from build123d import *

# Parameters (mm, degrees)
BOSS_EXTRUDE1_DEPTH  = 4
BOSS_EXTRUDE1_DRAFT  = -1
SHELL1_T             = -0.35
SKETCH2_W            = 12.58
SKETCH2_H            = 6.98
CUT_EXTRUDE1_DEPTH   = 2
SKETCH3_W            = 13.5
SKETCH3_H            = 13.096235698
CUT_EXTRUDE2_DEPTH   = 0.2
BOSS_EXTRUDE3_REACH  = 20.425
BOSS_EXTRUDE4_REACH  = 20.425
LPATTERN2_COUNT      = 2
LPATTERN2_PITCH      = 4
MIRROR4_COPY_1_REACH = 20.425
LPATTERN3_COUNT      = 2
LPATTERN3_PITCH      = 4
MIRROR5_COPY_1_REACH = 20.425
BOSS_EXTRUDE5_REACH  = 18.785
LPATTERN4_COUNT      = 2
LPATTERN4_PITCH      = 5
MIRROR6_COPY_1_REACH = 18.785
MIRROR6_COPY_2_REACH = 18.785


with BuildPart() as part:
    # Sketch1 → Boss-Extrude1 (with draft: the straight prism first)
    with BuildSketch(Plane(origin=(0, 0, 0), x_dir=(1, 0, 0), z_dir=(0, 1, 0))):
        with BuildLine():
            Line((-7.5, -8.5), (7.5, -8.5))
            ThreePointArc((7.5, -8.5), (8.207106781, -8.207106781), (8.5, -7.5))
            Line((8.5, -7.5), (8.5, 7.5))
            ThreePointArc((8.5, 7.5), (8.207106781, 8.207106781), (7.5, 8.5))
            Line((7.5, 8.5), (-7.5, 8.5))
            ThreePointArc((-7.5, 8.5), (-8.207106781, 8.207106781), (-8.5, 7.5))
            Line((-8.5, 7.5), (-8.5, -7.5))
            ThreePointArc((-8.5, -7.5), (-8.207106781, -8.207106781), (-7.5, -8.5))
        make_face()
    extrude(amount=-BOSS_EXTRUDE1_DEPTH)
    # Boss-Extrude1: the draft: its side faces are tilted about the plane it starts from
    boss_extrude1_sides = [part.faces().sort_by_distance(p)[0] for p in [
        (0, -2, 8.5),
        (8.207106781, -2, 8.207106781),
        (8.5, -2, 0),
        (8.207106781, -2, -8.207106781),
        (0, -2, -8.5),
        (-8.207106781, -2, -8.207106781),
        (-8.5, -2, 0),
        (-8.207106781, -2, 8.207106781),
    ]]
    draft(boss_extrude1_sides, Plane(origin=(0, 0, 0), x_dir=(1, 0, 0), z_dir=(0, 1, 0)), BOSS_EXTRUDE1_DRAFT)

    # Shell1
    shell1_openings = [part.faces().sort_by_distance(p)[0] for p in [
        (0, 0, 0),
    ]]
    offset(amount=SHELL1_T, openings=shell1_openings, kind=Kind.INTERSECTION)

    # Sketch2 → Cut-Extrude1 (cut)
    with BuildSketch(Plane.XZ.offset(4)):
        with Locations((0, 1.01)):
            Rectangle(SKETCH2_W, SKETCH2_H)
    extrude(amount=-CUT_EXTRUDE1_DEPTH, mode=Mode.SUBTRACT)

    # Sketch3 → Cut-Extrude2 (cut)
    with BuildSketch(Plane(origin=(0, -3.65, 0), x_dir=(1, 0, 0), z_dir=(0, 1, 0))):
        with Locations((0, 1.238117849)):
            Rectangle(SKETCH3_W, SKETCH3_H)
    extrude(amount=-CUT_EXTRUDE2_DEPTH, mode=Mode.SUBTRACT)

    # Boss-Extrude3: up to this plane
    boss_extrude3_end = Plane(origin=(8.150053307, 0.006108342, 7.5), z_dir=(0.9998476951563913, -0.01745240643728355, 0))
    # Sketch11 → Boss-Extrude3 (add, up to the surface)
    with BuildSketch(Plane.ZY.offset(-7.35), mode=Mode.PRIVATE) as boss_extrude3_sk1:
        Polygon((-0.455489584, -1.1), (0.46508987, -1.1), (0.509600286, -3.65), (-0.5, -3.65), align=None)
    boss_extrude3_tool1 = split(extrude(boss_extrude3_sk1.sketch, amount=-BOSS_EXTRUDE3_REACH, mode=Mode.PRIVATE), bisect_by=boss_extrude3_end, keep=Keep.BOTH, mode=Mode.PRIVATE)
    boss_extrude3 = boss_extrude3_tool1.solids().sort_by_distance((7.35, -2.394601, 0.0048))[0]
    add(boss_extrude3)

    # Boss-Extrude4: up to this plane
    boss_extrude4_end = Plane(origin=(-8.150053307, 0.006108342, 7.5), z_dir=(-0.9998476951563913, -0.01745240643728355, 0))
    # Sketch13 → Boss-Extrude4 (add, up to the surface)
    with BuildSketch(Plane(origin=(-7.35, 0, 0), x_dir=(0, 0, -1), z_dir=(1, 0, 0)), mode=Mode.PRIVATE) as boss_extrude4_sk1:
        Polygon((-0.5, -3.65), (0.509600286, -3.65), (0.46508987, -1.1), (-0.455489584, -1.1), align=None)
    boss_extrude4_tool1 = split(extrude(boss_extrude4_sk1.sketch, amount=-BOSS_EXTRUDE4_REACH, mode=Mode.PRIVATE), bisect_by=boss_extrude4_end, keep=Keep.BOTH, mode=Mode.PRIVATE)
    boss_extrude4 = boss_extrude4_tool1.solids().sort_by_distance((-7.35, -2.394601, -0.0048))[0]
    add(boss_extrude4)

    # LPattern2: Boss-Extrude3 ×2
    with Locations(*[(0, 0, i * LPATTERN2_PITCH) for i in range(1, LPATTERN2_COUNT)]):
        add(boss_extrude3)

    # Mirror4: Boss-Extrude3 across plane
    add(boss_extrude3.mirror(Plane.XY))

    # Mirror4 copy 1: up to this plane
    mirror4_copy_1_end = Plane(origin=(8.150053307, 0.006108342, 7.5), z_dir=(0.9998476951563913, -0.01745240643728355, 0))
    # Mirror4 copy 1 sketch → Mirror4 copy 1 (add, up to the surface)
    with BuildSketch(Plane(origin=(7.35, 0, -4), x_dir=(0, 0, -1), z_dir=(-1, 0, 0)), mode=Mode.PRIVATE) as mirror4_copy_1_sk1:
        Polygon((-0.455489584, 1.1), (0.46508987, 1.1), (0.509600286, 3.65), (-0.5, 3.65), align=None)
    mirror4_copy_1_tool1 = split(extrude(mirror4_copy_1_sk1.sketch, amount=-MIRROR4_COPY_1_REACH, mode=Mode.PRIVATE), bisect_by=mirror4_copy_1_end, keep=Keep.BOTH, mode=Mode.PRIVATE)
    add(mirror4_copy_1_tool1.solids().sort_by_distance((7.35, -2.394601, 0.0048))[0])

    # LPattern3: Boss-Extrude4 ×2
    with Locations(*[(0, 0, i * LPATTERN3_PITCH) for i in range(1, LPATTERN3_COUNT)]):
        add(boss_extrude4)

    # Mirror5: Boss-Extrude4 across plane
    add(boss_extrude4.mirror(Plane.XY))

    # Mirror5 copy 1: up to this plane
    mirror5_copy_1_end = Plane(origin=(-8.150053307, 0.006108342, 7.5), z_dir=(-0.9998476951563913, -0.01745240643728355, 0))
    # Mirror5 copy 1 sketch → Mirror5 copy 1 (add, up to the surface)
    with BuildSketch(Plane(origin=(-7.35, 0, -4), x_dir=(0, 0, 1), z_dir=(1, 0, 0)), mode=Mode.PRIVATE) as mirror5_copy_1_sk1:
        Polygon((-0.5, 3.65), (0.509600286, 3.65), (0.46508987, 1.1), (-0.455489584, 1.1), align=None)
    mirror5_copy_1_tool1 = split(extrude(mirror5_copy_1_sk1.sketch, amount=-MIRROR5_COPY_1_REACH, mode=Mode.PRIVATE), bisect_by=mirror5_copy_1_end, keep=Keep.BOTH, mode=Mode.PRIVATE)
    add(mirror5_copy_1_tool1.solids().sort_by_distance((-7.35, -2.394601, -0.0048))[0])

    # Boss-Extrude5: up to this plane
    boss_extrude5_end = Plane(origin=(-7.5, 0.006108342, 8.150053307), z_dir=(0, -0.017452406437283553, 0.9998476951563913))
    # Sketch16 → Boss-Extrude5 (add, up to the surface)
    with BuildSketch(Plane.XY.offset(5.41), mode=Mode.PRIVATE) as boss_extrude5_sk1:
        Polygon((-0.5, -3.65), (0.5, -3.65), (0.455489584, -1.1), (-0.455489584, -1.1), align=None)
    boss_extrude5_tool1 = split(extrude(boss_extrude5_sk1.sketch, amount=BOSS_EXTRUDE5_REACH, mode=Mode.PRIVATE), bisect_by=boss_extrude5_end, keep=Keep.BOTH, mode=Mode.PRIVATE)
    boss_extrude5 = boss_extrude5_tool1.solids().sort_by_distance((0, -2.394798, 5.41))[0]
    add(boss_extrude5)

    # LPattern4: Boss-Extrude5 ×2
    with Locations(*[(i * LPATTERN4_PITCH, 0, 0) for i in range(1, LPATTERN4_COUNT)]):
        add(boss_extrude5)

    # Mirror6 copy 1: up to this plane
    mirror6_copy_1_end = Plane(origin=(-7.5, 0.006108342, 8.150053307), z_dir=(0, -0.017452406437283553, 0.9998476951563913))
    # Mirror6 copy 1 sketch → Mirror6 copy 1 (add, up to the surface)
    with BuildSketch(Plane(origin=(-5, 0, 5.41), x_dir=(-1, 0, 0), z_dir=(0, 0, 1)), mode=Mode.PRIVATE) as mirror6_copy_1_sk1:
        Polygon((-0.5, 3.65), (0.5, 3.65), (0.455489584, 1.1), (-0.455489584, 1.1), align=None)
    mirror6_copy_1_tool1 = split(extrude(mirror6_copy_1_sk1.sketch, amount=MIRROR6_COPY_1_REACH, mode=Mode.PRIVATE), bisect_by=mirror6_copy_1_end, keep=Keep.BOTH, mode=Mode.PRIVATE)
    add(mirror6_copy_1_tool1.solids().sort_by_distance((0, -2.394798, 5.41))[0])

    # Mirror6 copy 2: up to this plane
    mirror6_copy_2_end = Plane(origin=(-7.5, 0.006108342, 8.150053307), z_dir=(0, -0.017452406437283553, 0.9998476951563913))
    # Mirror6 copy 2 sketch → Mirror6 copy 2 (add, up to the surface)
    with BuildSketch(Plane(origin=(0, 0, 5.41), x_dir=(-1, 0, 0), z_dir=(0, 0, 1)), mode=Mode.PRIVATE) as mirror6_copy_2_sk1:
        Polygon((-0.5, 3.65), (0.5, 3.65), (0.455489584, 1.1), (-0.455489584, 1.1), align=None)
    mirror6_copy_2_tool1 = split(extrude(mirror6_copy_2_sk1.sketch, amount=MIRROR6_COPY_2_REACH, mode=Mode.PRIVATE), bisect_by=mirror6_copy_2_end, keep=Keep.BOTH, mode=Mode.PRIVATE)
    add(mirror6_copy_2_tool1.solids().sort_by_distance((0, -2.394798, 5.41))[0])

    # Sweep1: sweep along a path in Sketch18
    with BuildLine(Plane(origin=(0, -2, 0), x_dir=(-1, 0, 0), z_dir=(0, -1, 0))) as sweep1_path:
        Line((8.5, 7.5), (8.5, -7.5))
        ThreePointArc((8.5, -7.5), (8.207106781, -8.207106781), (7.5, -8.5))
        Line((7.5, -8.5), (-7.5, -8.5))
        ThreePointArc((-7.5, -8.5), (-8.207106781, -8.207106781), (-8.5, -7.5))
        Line((-8.5, -7.5), (-8.5, 7.5))
        ThreePointArc((-8.5, 7.5), (-8.207106781, 8.207106781), (-7.5, 8.5))
        Line((-7.5, 8.5), (7.5, 8.5))
        ThreePointArc((7.5, 8.5), (8.207106781, 8.207106781), (8.5, 7.5))
    # Sketch17 → Sweep1 (sweep)
    with BuildSketch(Plane.XY):
        Polygon((-8.5, 0), (-8.46508987, -2), (-8.76508987, -2), align=None)
    sweep(path=sweep1_path.line)

    # Sweep2: sweep along a path in Sketch23
    with BuildLine(Plane(origin=(0, 0, 0), x_dir=(1, 0, 0), z_dir=(0, 1, 0))) as sweep2_path:
        Line((8.149946685, -7.5), (8.149946685, 7.5))
        ThreePointArc((8.149946685, 7.5), (7.959581709, 7.959581709), (7.5, 8.149946685))
        Line((7.5, 8.149946685), (-7.5, 8.149946685))
        ThreePointArc((-7.5, 8.149946685), (-7.959581709, 7.959581709), (-8.149946685, 7.5))
        Line((-8.149946685, 7.5), (-8.149946685, -7.5))
        ThreePointArc((-8.149946685, -7.5), (-7.959581709, -7.959581709), (-7.5, -8.149946685))
        Line((-7.5, -8.149946685), (7.5, -8.149946685))
        ThreePointArc((7.5, -8.149946685), (7.959581709, -7.959581709), (8.149946685, -7.5))
    # Sketch19 → Sweep2 (sweep)
    with BuildSketch(Plane.XY):
        Polygon((8.149946685, 0), (8.148156734, -0.102546259), (8.14097505, -0.102546259), align=None)
    sweep(path=sweep2_path.line)


solid = part.part
Could you check a few things on this model? Use its own coordinates, in mm. A direction names the side the tool comes from. Coordinates: 2 decimals unless noted, no trailing zeros. Order: outer loops, then holes, each group sorted by start corner. A loop starts at its lowest first (then second) coordinate and runs counter-clockwise, first axis right, second up. Notation, with made-up numbers: (-24, 37) - (24, 37) arc R16 ccw to (24, 49) - close; hole circle Ø5 at (44.25, -13). An arc over 180 degrees is marked (long way). Answer in a Markdown table with one row per item. Add a question column.
(1) I need wall thicknesses on L1, parallel to Z at x = -8, y = -1.4; L2, parallel to Z at x = 1.25, y = -2.5; L3, parallel to Y at x = 5.75, z = 6.5. Which ranges of each line are inside material? Lowest first, please.
(2) Will these pins go through, and if not, where does the flat tip stop? pin 1 (2 mm diameter, centred on x = 3.5, z = 2.5, fed in from -Y); pin 2 (1.5 mm diameter, centred on x = -7, y = -3.5, fed in from -Z); pin 3 (6.5 mm diameter, centred on x = -2, z = 0, fed in from +Y); pin 4 (2 mm diameter, centred on y = -0.5, z = 2, fed in from -X).
(3) If we mould it in two halves opening along Z, with no side actions, what happens to faces 1 (the face through (0.1, -0.99, 8.63)), 2 (the face through (8.18, -2.99, -8.16)), 3 (the face through (-7.35, -2, 0))? For each: released by +Z, released by -Z, zero draft, split by the parting line, or undercut.
(4) If we section it at C-C, the plane y = -0.7: Please give me the cut outline in (x, z).
(5) On a 3-axis mill with a long thin cutter (end or side, diameter ignored), from which of +Z, -Z, +X, -X, +Y, -Y can I reach the whole of each face in a straight line? I mean faces 4 (the face through (5, -2, 5.41)), 5 (the face through (-8.3, -1, -8.3)). Say none if no direction works.
Results are:
| question | item | result |
|---|---|---|
| 1 | L1 | z = -8.57 to -7.88, -4.46 to -3.53, -0.47 to 0.47, 3.53 to 4.46, 7.88 to 8.57 |
| 1 | L2 | z = -8.46 to -8.11, 8.11 to 8.46 |
| 1 | L3 | y = -4 to -3.65 |
| 2 | pin 1 | passes through |
| 2 | pin 2 | stops at z = -8.45 |
| 2 | pin 3 | stops at y = -3.85 |
| 2 | pin 4 | stops at x = -8.7 |
| 3 | face 1 | released by +Z |
| 3 | face 2 | released by -Z |
| 3 | face 3 | undercut |
| 4 | outline | (-8.59, -7.5) arc R1.09 ccw to (-7.5, -8.59) - (7.5, -8.59) arc R1.09 ccw to (8.59, -7.5) - (8.59, 7.5) arc R1.09 ccw to (7.5, 8.59) - (-7.5, 8.59) arc R1.09 ccw to (-8.59, 7.5) - close; hole (-8.14, -7.5) arc R0.64 ccw to (-7.5, -8.14) - (7.5, -8.14) arc R0.64 ccw to (8.14, -7.5) - (8.14, 7.5) arc R0.64 ccw to (7.5, 8.14) - (-7.5, 8.14) arc R0.64 ccw to (-8.14, 7.5) - close |
| 5 | face 4 | +Y |
| 5 | face 5 | -Z, -X, +Y |
